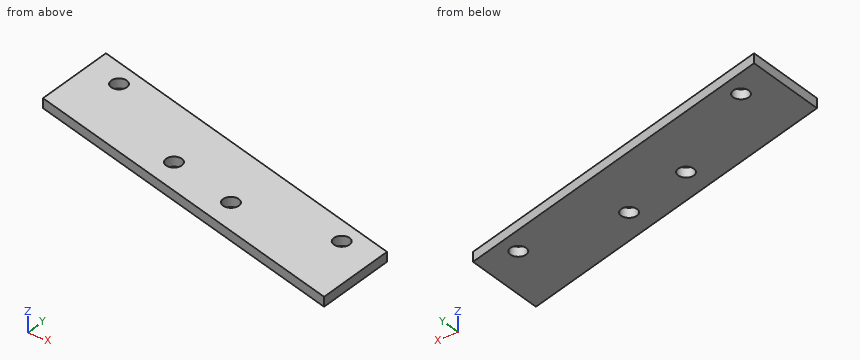
from build123d import *

# Parameters (mm, degrees)
RESSALTO_EXTRUS_O1_DEPTH                = 3
BROCA_DE_ROSQUEAR_PARA_TARRAXA_DE_M61_D = 5


with BuildPart() as part:
    # Esboço1 → Ressalto-extrusão1 (new body)
    with BuildSketch(Plane.XY):
        Polygon((0, 0), (0, 25.814370739), (110.897531805, -2.721177961), (110.897531805, -28.5355487), align=None)
    extrude(amount=RESSALTO_EXTRUS_O1_DEPTH)

    # Broca de rosquear para tarraxa de M61 (through all)
    with Locations(Plane.XY.offset(3)):
        with Locations((11.117838312, 16.758140178), (43.720802317, -2.989400019), (66.208276673, -8.775754406), (98.985562185, -5.851503814)):
            Hole(BROCA_DE_ROSQUEAR_PARA_TARRAXA_DE_M61_D / 2)


solid = part.part
The model under review builds one solid part; all positions refer to its coordinate system, in mm. Round coordinates to 2 decimals unless told otherwise and drop trailing zeros. Write each loop counter-clockwise with the first axis right and the second up, starting at its lowest first coordinate (ties: lowest second). Pieces come first, ordered by that corner, then holes. Notation, with made-up numbers: (35, -10) - (72, -10) arc R30 ccw to (72, 21) - close; hole circle Ø5 at (48, -39). An arc over 180 degrees is marked (long way). One line per item, written item: value. Start each with the question number.
1. Consider section B-B on y = -24. Write out the cut boundary in (x, z), and give its area (3 significant figures).
2. Consider section C-C on x = 79. Write out the cut boundary in (y, z), and give its area (3 significant figures).
3. Consider section A-A on z = 0.55. Write out the cut boundary in (x, y), and give its area (3 significant figures).
4. To check wall thickness, follow L1, parallel to Y at x = 9, z = 1.5; L2, parallel to Y at x = 46, z = 1.2; L3, parallel to Y at x = 36, z = 0.3. State the ranges of each line that lie inside material, in increasing order. Write a range as from..to.
Checks:
1. outline: (93.27, 0) - (110.9, 0) - (110.9, 3) - (93.27, 3) - close
1. area: 52.9 mm^2
2. outline: (-20.33, 0) - (5.49, 0) - (5.49, 3) - (-20.33, 3) - close
2. area: 77.4 mm^2
3. outline: (0, 0) - (110.9, -28.54) - (110.9, -2.72) - (0, 25.81) - close; hole circle Ø5 at (11.12, 16.76); hole circle Ø5 at (43.72, -2.99); hole circle Ø5 at (66.21, -8.78); hole circle Ø5 at (98.99, -5.85)
3. area: 2,780 mm^2
4. L1: y = -2.32..15.43, 18.09..23.5
4. L2: y = -11.84..-4.02, -1.96..13.98
4. L3: y = -9.26..16.55
